```python
from build123d import *

# Parameters (mm, degrees)
F0_R     = 2
F1_DEPTH = 5
F2_DEPTH = 45
F3_DEPTH = 5
F4_DEPTH = 5
F5_R     = 4.99999


# Not quite as in the source:
# - a fillet or chamfer is up to 0.001 mm smaller than in the source, because OpenCascade refuses the exact size


with BuildPart() as f1:
    # F0 (on Top) → F1 (new body)
    with BuildSketch(Plane.XY):
        Polygon((-17.7, 22.7), (-17.7, 0), (-17.7, -22.7), (27.7, -22.7), (27.7, 22.7), align=None)
        with Locations((22.7, -17.7)):
            Circle(F0_R, mode=Mode.SUBTRACT)
        with BuildLine():
            ThreePointArc((-17.7, 0), (0, 17.7), (17.7, 0))
            ThreePointArc((17.7, 0), (0, -17.7), (-17.7, 0))
        make_face(mode=Mode.SUBTRACT)
        with Locations((22.7, 17.7)):
            Circle(F0_R, mode=Mode.SUBTRACT)
        with BuildLine():
            ThreePointArc((-17.7, 0), (0, -17.7), (17.7, 0))
            ThreePointArc((17.7, 0), (0, 17.7), (-17.7, 0))
        make_face()
    extrude(amount=F1_DEPTH)

    # F0 (on Top) → F2 (join)
    with BuildSketch(Plane.XY):
        with BuildLine():
            ThreePointArc((-17.7, 0), (0, -17.7), (17.7, 0))
            ThreePointArc((17.7, 0), (0, 17.7), (-17.7, 0))
        make_face()
    extrude(amount=F2_DEPTH)

    # F0 (on Top) → F3 (join, through all)
    with BuildSketch(Plane.XY):
        Polygon((-17.7, -22.7), (-17.7, 0), (-17.7, 22.7), (-27.7, 22.7), (-27.7, -22.7), align=None)
    extrude(amount=F3_DEPTH)

    # F0 (on Top) → F4 (join)
    with BuildSketch(Plane.XY):
        Polygon((-17.7, -22.7), (-17.7, 0), (-17.7, 22.7), (-27.7, 22.7), (-27.7, -22.7), align=None)
    extrude(amount=-F4_DEPTH)

    # F5 (radius 5 in the source; OpenCascade refuses exactly that, so slightly less here)
    f5_edges = [f1.edges().sort_by_distance(p)[0] for p in [
        (-17.7, 0, 5),
    ]]
    fillet(f5_edges, radius=F5_R)


solid = f1.part
```
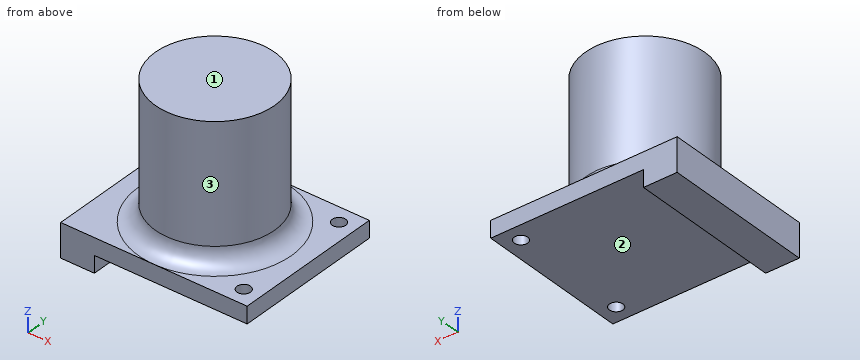
Could you check a few things on this model? Use its own coordinates, in mm. Face numbers are marked on the shaded views. A direction names the side the tool comes from. Give positions to 0.01 mm unless a question says otherwise; leave off trailing zeros. Write each loop counter-clockwise with the first axis right and the second up, starting at its lowest first coordinate (ties: lowest second). Pieces come first, ordered by that corner, then holes. Notation, with made-up numbers: (58, 21.5) -> (79, 21.5) arc R27 ccw to (79, 41.5) -> close; hole circle Ø11 at (85.5, 76.25). An arc over 180 degrees is marked (long way). Write each question's results on one line, items separated by ' | '.
1. On a 3-axis mill with a long thin cutter (end or side, diameter ignored), from which of +Z, -Z, +X, -X, +Y, -Y can I reach the whole of each face in a straight line? I mean the marked faces 1, 2 and 3. Say none if no direction works.
Check sheet entries:
face 1: +Z, +X, -X, +Y, -Y | face 2: -Z, +X, +Y, -Y | face 3: +Z
2. Will these pins go through, and if not, where does the flat tip stop? pin 1 Ø5 at (y, z) = (1, 14.5) entering from -X; pin 2 Ø6 at (x, z) = (14, 34) entering from +Y; pin 3 Ø2 at (x, z) = (20.5, 27.5) entering from -Y; pin 4 Ø6 at (x, z) = (1.5, 19) entering from -Y.
Check sheet entries:
pin 1: stops at x = -17.7 | pin 2: stops at y = 13.87 | pin 3: passes through | pin 4: stops at y = -17.7
3. I want a section at B-B, the plane y = 0. Write out the boundary of the cut face in (x, z), then the cut area to 3 significant figures.
Check sheet entries:
outline: (-27.7, -5) -> (-17.7, -5) -> (-17.7, 0) -> (27.7, 0) -> (27.7, 5) -> (22.7, 5) arc R5 cw to (17.7, 10) -> (17.7, 45) -> (-17.7, 45) -> (-17.7, 10) arc R5 cw to (-22.7, 5) -> (-27.7, 5) -> close | area: 1,750 mm²
4. I want a section at C-C, the plane z = 7. Write out the boundary of the cut face in (x, y), then the cut area to 3 significant figures.
Check sheet entries:
outline: circle Ø37.4 at (0, 0) | area: 1,100 mm²
5. I need wall thicknesses on L1, parallel to Y at x = 22.7, z = 1.35; L2, parallel to Y at x = 22, z = 1; L3, parallel to Z at x = 13, y = 19. Which ranges of each line are inside material? Lowest first, please.
Check sheet entries:
L1: y = -22.7 to -19.7, -15.7 to 15.7, 19.7 to 22.7 | L2: y = -22.7 to -19.57, -15.83 to 15.83, 19.57 to 22.7 | L3: z = 0 to 5
